from build123d import *

# Parameters (mm, degrees)
BOSS_EXTRUDE1_DEPTH = 8
FILLET1_R           = 4
FILLET2_R           = 4
FILLET3_R           = 4
SKETCH2_R           = 2
CUT_EXTRUDE1_DEPTH  = 20.595917942


with BuildPart() as part:
    # Sketch1 → Boss-Extrude1 (new body)
    with BuildSketch(Plane(origin=(0, 0, 0), x_dir=(1, 0, 0), z_dir=(0, 1, 0))):
        with BuildLine():
            Line((0, 0), (0, 12))
            ThreePointArc((0, 12), (-3.2, 15.2), (-6.4, 12))
            Line((-6.4, 12), (-6.4, 0))
            Line((-6.4, 0), (-7.2, 0))
            Line((-7.2, 0), (-7.2, 12))
            ThreePointArc((-7.2, 12), (-3.2, 16), (0.8, 12))
            Line((0.8, 12), (0.8, 0))
            Line((0.8, 0), (0, 0))
        make_face()
    extrude(amount=BOSS_EXTRUDE1_DEPTH)

    # Fillet1
    fillet1_edges = [part.edges().sort_by_distance(p)[0] for p in [
        (0.4, 8, 0),
    ]]
    fillet(fillet1_edges, radius=FILLET1_R)

    # Fillet2
    fillet2_edges = [part.edges().sort_by_distance(p)[0] for p in [
        (0.4, 0, 0),
    ]]
    fillet(fillet2_edges, radius=FILLET2_R - 0.0001)  # a hair under: the kernel refuses the full size

    # Fillet3
    fillet3_edges = [part.edges().sort_by_distance(p)[0] for p in [
        (-6.8, 0, 0),
        (-6.8, 8, 0),
    ]]
    fillet(fillet3_edges, radius=FILLET3_R - 0.0001)  # a hair under: the kernel refuses the full size

    # Sketch2 → Cut-Extrude1 (cut, through all)
    with BuildSketch(Plane(origin=(0.8, 0, 0), x_dir=(0, 0, -1), z_dir=(1, 0, 0))):
        with Locations((4, 4)):
            Circle(SKETCH2_R)
    extrude(amount=-CUT_EXTRUDE1_DEPTH, mode=Mode.SUBTRACT)


solid = part.part
Design review of the part built by this model. Coordinates are the model's own, in mm. A direction names the side the tool comes from. Coordinates: 2 decimals unless noted, no trailing zeros. Order: outer loops, then holes, each group sorted by start corner. A loop starts at its lowest first (then second) coordinate and runs counter-clockwise, first axis right, second up.
Item 1: The part is to be moulded in two halves that separate along Z. For faces 1 (the cylindrical face through (0.394, 1.203, -1.141)), 2 (the flat face through (0, 4, -7)), 3 (the cylindrical face through (-6.8, 2.8, -2.4)), say which applies: pulls with the +Z half, pulls with the -Z half, needs draft (parallel to the pull), parting line crosses it, or undercut.
Item 2: Take a section at D-D, the plane z = -5. Write out the cut boundary in (x, y).
Item 3: Take a section at A-A, the plane z = -9.75. Write out the cut boundary in (x, y).
Item 4: For pin 1 Ø2 at (x, y) = (-3, 6.5) entering from +Z; pin 2 Ø4 at (x, y) = (-6.5, 3) entering from +Z, all flat-tipped, find the tip position at first contact; note any pin that passes through.
Item 5: For line 1 (X direction, y = 1.75, z = -7.75); line 2 (Y direction, x = -6.6, z = -4); line 3 (X direction, y = 3, z = -13), list the stretches that pass through material, from the lowest coordinate up.
Item 6: Take a section at B-B, the plane y = 3.25. Write out the cut boundary in (x, z).
Item 7: For faces 4 (the cylindrical face through (-6.806, 6.859, -1.203)), 5 (the flat face through (-6.4, 4, -7)), list the 3-axis set-ups (+Z, -Z, +X, -X, +Y, -Y) from which the entire face can be reached by the end or side of a thin tool; tool diameter is ignored.
The answers:
1. face 1: pulls with the +Z half
1. face 2: needs draft
1. face 3: undercut
2. outline: (-7.2, 0) - (-6.4, 0) - (-6.4, 2.27) - (-7.2, 2.27) - close; (-7.2, 5.73) - (-6.4, 5.73) - (-6.4, 8) - (-7.2, 8) - close; (0, 0) - (0.8, 0) - (0.8, 2.27) - (0, 2.27) - close; (0, 5.73) - (0.8, 5.73) - (0.8, 8) - (0, 8) - close
3. outline: (-7.2, 0) - (-6.4, 0) - (-6.4, 8) - (-7.2, 8) - close; (0, 0) - (0.8, 0) - (0.8, 8) - (0, 8) - close
4. pin 1: stops at z = -14.97
4. pin 2: stops at z = 0
5. line 1: x = -7.2 to -6.4, 0 to 0.8
5. line 2: y = 0 to 2, 6 to 8
5. line 3: x = -7.07 to -6.24, -0.16 to 0.67
6. outline: (-7.2, -12) arc R4 ccw to (0.8, -12) - (0.8, -5.85) - (0, -5.85) - (0, -12) arc R3.2 cw to (-6.4, -12) - (-6.4, -5.85) - (-7.2, -5.85) - close; (-7.2, -2.15) - (-6.4, -2.15) - (-6.4, -0.07) - (-7.2, -0.07) - close; (0, -2.15) - (0.8, -2.15) - (0.8, -0.07) - (0, -0.07) - close
7. face 4: +Z, +X, -X, +Y
7. face 5: +Z, +Y, -Y
